```python
from build123d import *

# Parameters (mm, degrees)
SKETCH1_W           = 151.765
SKETCH1_H           = 177.165
BOSS_EXTRUDE1_DEPTH = 19.05


with BuildPart() as part:
    # Sketch1 → Boss-Extrude1 (new body)
    with BuildSketch(Plane(origin=(0, -0.635, 0), x_dir=(-1, 0, 0), z_dir=(0, -1, 0))):
        Rectangle(SKETCH1_W, SKETCH1_H)
        with BuildLine():
            Line((13.6525, 26.67), (13.6525, 82.55))
            Line((13.6525, 82.55), (-63.5, 82.55))
            ThreePointArc((-63.5, 82.55), (-67.990128061, 80.690128061), (-69.85, 76.2))
            Line((-69.85, 76.2), (-69.85, 33.02))
            ThreePointArc((-69.85, 33.02), (-67.990128061, 28.529871939), (-63.5, 26.67))
            Line((-63.5, 26.67), (13.6525, 26.67))
        make_face(mode=Mode.SUBTRACT)
        with BuildLine():
            Line((13.6525, -82.55), (13.6525, -26.67))
            Line((13.6525, -26.67), (-63.5, -26.67))
            ThreePointArc((-63.5, -26.67), (-67.990128061, -28.529871939), (-69.85, -33.02))
            Line((-69.85, -33.02), (-69.85, -76.2))
            ThreePointArc((-69.85, -76.2), (-67.990128061, -80.690128061), (-63.5, -82.55))
            Line((-63.5, -82.55), (13.6525, -82.55))
        make_face(mode=Mode.SUBTRACT)
        with BuildLine():
            Line((7.3025, -19.05), (-63.5, -19.05))
            ThreePointArc((-63.5, -19.05), (-67.990128061, -17.190128061), (-69.85, -12.7))
            Line((-69.85, -12.7), (-69.85, 12.7))
            ThreePointArc((-69.85, 12.7), (-67.990128061, 17.190128061), (-63.5, 19.05))
            Line((-63.5, 19.05), (7.3025, 19.05))
            ThreePointArc((7.3025, 19.05), (11.792628061, 17.190128061), (13.6525, 12.7))
            Line((13.6525, 12.7), (13.6525, -12.7))
            ThreePointArc((13.6525, -12.7), (11.792628061, -17.190128061), (7.3025, -19.05))
        make_face(mode=Mode.SUBTRACT)
        with BuildLine():
            Line((29.5275, -82.55), (60.0075, -82.55))
            ThreePointArc((60.0075, -82.55), (66.742692091, -79.760192091), (69.5325, -73.025))
            Line((69.5325, -73.025), (69.5325, 73.025))
            ThreePointArc((69.5325, 73.025), (66.742692091, 79.760192091), (60.0075, 82.55))
            Line((60.0075, 82.55), (29.5275, 82.55))
            ThreePointArc((29.5275, 82.55), (22.792307909, 79.760192091), (20.0025, 73.025))
            Line((20.0025, 73.025), (20.0025, -73.025))
            ThreePointArc((20.0025, -73.025), (22.792307909, -79.760192091), (29.5275, -82.55))
        make_face(mode=Mode.SUBTRACT)
    extrude(amount=BOSS_EXTRUDE1_DEPTH)


solid = part.part
```
For this review, take the finished solid that the model builds, in its own axes (mm). A direction names the side the tool comes from. Give positions to 0.01 mm unless a question says otherwise; leave off trailing zeros. Answer as a JSON object with one key per item and string values. Group by question number.
Item 1: Tool access review of faces 4 (the cylindrical face through (68.04, -10.03, -17.14)), 5 (the flat face through (6, -0.635, 19.3)): name each direction out of +Z, -Z, +X, -X, +Y, -Y from which nothing blocks a thin tool from reaching the whole face with its end or side.
Item 2: Draft analysis for pull direction Z (two halves, no side actions). For faces 1 (the flat face through (75.882, -10, 1)), 2 (the flat face through (25, -10, -26.67)), 3 (the flat face through (1, -10, 88.582)), state which applies: +Z half, -Z half, draft (parallel to the pull), parting line (faces both ways), or undercut.
Item 3: For pin 1 Ø3 at (x, z) = (24.5, 17.5) entering from -Y; pin 2 Ø10 at (x, z) = (48, 29) entering from -Y (3 decimals), all flat-tipped, find the tip position at first contact; note any pin that passes through.
Item 4: For probe 1 along Z at (x, y) = (37, -5.75); probe 2 along X at (y, z) = (-14.5, -32.5); probe 3 along Z at (x, y) = (-32, -12.5), list the stretches that pass through material, from the lowest coordinate up. Write a range as [from, to].
Item 5: Consider section A-A on x = 5. Count the separate pieces of the cut face and the enclosed holes in it, plus the area to 3 significant figures.
Check result:
{
 "1": {"face 4": "+Y, -Y", "face 5": "+Z, -Z, +X, -X, +Y"},
 "2": {"face 1": "draft", "face 2": "undercut", "face 3": "+Z half"},
 "3": {"pin 1": "passes through", "pin 2": "stops at y = -19.685"},
 "4": {"probe 1": "z = [-88.58, -82.55], [-26.67, -19.05], [19.05, 26.67], [82.55, 88.58]", "probe 2": "x = [-75.88, -69.53], [-20, -13.65], [69.83, 75.88]", "probe 3": "z = [-88.58, -82.55], [82.55, 88.58]"},
 "5": {"separate pieces": "4", "enclosed holes": "0", "area": "520 mm^2"}
}
